from build123d import *
from OCP.BRepAlgoAPI import BRepAlgoAPI_Cut
from OCP.TopTools import TopTools_ListOfShape

# Parameters (mm, degrees)
SKETCH1_R                = 5
BOSS_EXTRUDE1_DEPTH      = 40
SKETCH2_R                = 5
BOSS_EXTRUDE2_DEPTH      = 20
SKETCH4_R                = 5
BOSS_EXTRUDE3_DEPTH      = 20
BOSS_EXTRUDE4_DEPTH      = 10
BOSS_EXTRUDE4_DEPTH_BACK = 13.827204
SKETCH6_R                = 5
SKETCH8_R                = 5
CUT_EXTRUDE1_DEPTH       = 3.827204
SKETCH13_R               = 5
BOSS_EXTRUDE5_DEPTH      = 20
SKETCH14_R               = 3
CUT_EXTRUDE2_DEPTH       = 12
CUT_EXTRUDE3_START       = -12
SKETCH15_R               = 3
CUT_EXTRUDE3_DEPTH       = 12
SKETCH16_R               = 3
CUT_EXTRUDE4_DEPTH       = 12
SKETCH17_R               = 3
CUT_EXTRUDE5_DEPTH       = 12
SKETCH18_R               = 3
CUT_EXTRUDE6_DEPTH       = 12
SKETCH19_R               = 3
CUT_EXTRUDE7_DEPTH       = 12


with BuildPart() as part:
    # Sketch1 → Boss-Extrude1 (new body)
    with BuildSketch(Plane(origin=(0, 0, 0), x_dir=(1, 0, 0), z_dir=(0, 1, 0))):
        with Locations(Location((0, 0, 0), (0, 0, 270))):
            Circle(SKETCH1_R)
    extrude(amount=BOSS_EXTRUDE1_DEPTH)

    # Sketch2 → Boss-Extrude2 (add)
    with BuildSketch(Plane.XY):
        with Locations((0, 20)):
            Circle(SKETCH2_R)
    extrude(amount=BOSS_EXTRUDE2_DEPTH)

    # Sketch4 → Boss-Extrude3 (add)
    with BuildSketch(Plane(origin=(0, 10, -10), x_dir=(-1, 0, 0), z_dir=(0, -0.7071067811865475, 0.7071067811865477))):
        with Locations(Location((0, -14.142135624, 0), (0, 0, 90))):
            Circle(SKETCH4_R)
    extrude(amount=BOSS_EXTRUDE3_DEPTH)

    # Sketch6 → Boss-Extrude4 (add, two sides: drawn at the far end of the back side and taken through both)
    with BuildSketch(Plane(origin=(11.97471023, 0, 6.913602175), x_dir=(0.49999999999999756, 0, -0.86602540378444), z_dir=(0.86602540378444, 0, 0.49999999999999756)).offset(-BOSS_EXTRUDE4_DEPTH_BACK)):
        with Locations((0, 20)):
            Circle(SKETCH6_R)
    extrude(amount=BOSS_EXTRUDE4_DEPTH + BOSS_EXTRUDE4_DEPTH_BACK)

    # Sketch8 → Cut-Extrude1 (cut)
    with BuildSketch(Plane(origin=(20.634964268, 0, 11.913602175), x_dir=(0.49999999999999756, 0, -0.86602540378444), z_dir=(0.86602540378444, 0, 0.49999999999999756))):
        with Locations((0, 20)):
            Circle(SKETCH8_R)
    extrude(amount=-CUT_EXTRUDE1_DEPTH, mode=Mode.SUBTRACT)

    # Sketch13 → Boss-Extrude5 (add)
    with BuildSketch(Plane(origin=(8.660254038, 10, 5), x_dir=(0.7905694150420939, -0.5477225575051677, -0.2738612787525826), z_dir=(0.6123724356957958, 0.7071067811865471, 0.3535533905932725))):
        with Locations(Location((-10.95445115, 8.94427191, 0), (0, 0, 50.768479516))):
            Circle(SKETCH13_R)
    extrude(amount=BOSS_EXTRUDE5_DEPTH)

    # Sketch14 → Cut-Extrude2 (cut)
    with BuildSketch(Plane(origin=(0, 40, 0), x_dir=(1, 0, 0), z_dir=(0, 1, 0))):
        with Locations(Location((0, 0, 0), (0, 0, 270))):
            Circle(SKETCH14_R)
    extrude(amount=-CUT_EXTRUDE2_DEPTH, mode=Mode.SUBTRACT)

    # Sketch15 → Cut-Extrude3 (cut)
    with BuildSketch(Plane.XZ.offset(CUT_EXTRUDE3_START)):
        with Locations(Location((0, 0, 0), (0, 0, 90))):
            Circle(SKETCH15_R)
    extrude(amount=CUT_EXTRUDE3_DEPTH, mode=Mode.SUBTRACT)

    # Sketch16 → Cut-Extrude4 (cut)
    with BuildSketch(Plane(origin=(0, -4.142135624, 4.142135624), x_dir=(1, 0, 0), z_dir=(0, -0.7071067811865476, 0.7071067811865476))):
        with Locations(Location((0, 14.142135624, 0), (0, 0, 270))):
            Circle(SKETCH16_R)
    extrude(amount=-CUT_EXTRUDE4_DEPTH, mode=Mode.SUBTRACT)

    # Sketch17 → Cut-Extrude5 (cut)
    with BuildSketch(Plane.XY.offset(20)):
        with Locations((0, 20)):
            Circle(SKETCH17_R)
    extrude(amount=-CUT_EXTRUDE5_DEPTH, mode=Mode.SUBTRACT)


with BuildPart() as cut_extrude6_tool:
    # Sketch18 → Cut-Extrude6 (new body)
    with BuildSketch(Plane(origin=(17.320508076, 0, 10), x_dir=(0.49999999999999756, 0, -0.86602540378444), z_dir=(0.86602540378444, 0, 0.49999999999999756))):
        with Locations((0, 20)):
            Circle(SKETCH18_R)
    extrude(amount=-CUT_EXTRUDE6_DEPTH)


with BuildPart() as part_1:
    add(part.part)

    # Cut-Extrude6: cut by cut_extrude6_tool, with a tolerance
    cut_extrude6_stock = TopTools_ListOfShape()
    cut_extrude6_stock.Append(part_1.part.wrapped)
    cut_extrude6_tools = TopTools_ListOfShape()
    cut_extrude6_tools.Append(cut_extrude6_tool.part.wrapped)
    cut_extrude6_cut = BRepAlgoAPI_Cut()
    cut_extrude6_cut.SetArguments(cut_extrude6_stock)
    cut_extrude6_cut.SetTools(cut_extrude6_tools)
    cut_extrude6_cut.SetFuzzyValue(0.00001)
    cut_extrude6_cut.Build()
    add(Compound.cast(cut_extrude6_cut.Shape()).solids(), mode=Mode.REPLACE)

    # Sketch19 → Cut-Extrude7 (cut)
    with BuildSketch(Plane(origin=(20.907702752, 24.142135624, 12.071067812), x_dir=(0.7905694150420939, -0.5477225575051676, -0.273861278752583), z_dir=(0.6123724356957958, 0.7071067811865471, 0.35355339059327245))):
        with Locations(Location((-10.95445115, 8.94427191, 0), (0, 0, 162.976133815))):
            Circle(SKETCH19_R)
    extrude(amount=-CUT_EXTRUDE7_DEPTH, mode=Mode.SUBTRACT)


solid = part_1.part
Model file for the job. Use its own axes, mm. A direction names the side the tool comes from. Give positions to 0.01 mm unless a question says otherwise; leave off trailing zeros. Write item = value, one per line. Start each with the question number.
1. Probe line 1 along X through (y, z) = (33.25, 0); line 2 along Y through (x, z) = (7, 4.75); line 3 along Y through (x, z) = (-1.25, 16). List the from-to ranges inside material, lowest first.
2. Cut at A-A, the plane y = 6. State how many separate pieces and enclosed holes the cut face has, and give its area (3 significant figures).
3. Drop flat-ended pins along their axis: P1, Ø5, axis at y = 11, z = 11, coming from the +X side; P2, Ø1.8, axis at x = -1.5, y = 19, coming from the +Z side; P3, Ø2, axis at y = 11.5, z = 11.5, coming from the -X side; P4, Ø1.5, axis at x = 16.5, y = 13, coming from the +Z side. Give the stop position or say it passes through.
4. Two-plate mould, pull along X, no slides. Class faces 5 (the flat face through (-3.3, 40, -0.1)), 6 (the cylindrical face through (-0.65, 17.07, 14.08)), 7 (the flat face through (17.286, 16.737, 10.061)): pulls with the +X half, pulls with the -X half, needs draft (parallel to the pull), parting line crosses it, or undercut.
5. Which spindle directions (+Z, -Z, +X, -X, +Y, -Y) get a long thin tool onto all of the face, cutting with end or side? Do faces 1 (the flat face through (0, 12, 0)), 2 (the cylindrical face through (0.9, 34.08, 2.86)), 3 (the cylindrical face through (-3, 20, -4)), 4 (the flat face through (0, 20, 8)). Say none if no direction does.
Taken from the geometry:
q1.line_1 = -5 to -3, 3 to 5
q1.line_2 = 15.04 to 17.06, 22.94 to 24.28, 32.59 to 35.45
q1.line_3 = 7.86 to 10.85, 15.16 to 17.27, 22.73 to 24.84
q2.separate_pieces = 2
q2.enclosed_holes = 1
q2.area = 86.9 mm²
q3.P1 = 5
q3.P2 = 8
q3.P3 = -4.87
q3.P4 = through
q4.face_5 = needs draft
q4.face_6 = undercut
q4.face_7 = pulls with the +X half
q5.face_1 = -Y
q5.face_2 = +Y
q5.face_3 = none
q5.face_4 = +Z
